```python
from build123d import *

# Parameters (mm, degrees)
BOSS_EXTRUDE1_DEPTH = 1.27
SKETCH2_R           = 2.0955
CUT_EXTRUDE1_DEPTH  = 2.27
CUT_EXTRUDE2_DEPTH  = 12.233456041


with BuildPart() as part:
    # Sketch1 → Boss-Extrude1 (new body)
    with BuildSketch(Plane.XY):
        with BuildLine():
            Line((48.63672497, 40.016070461), (47.23972497, 17.664070461))
            Line((47.23972497, 17.664070461), (45.08072497, 17.664070461))
            Line((45.08072497, 17.664070461), (45.138829135, 14.362070461))
            ThreePointArc((45.138829135, 14.362070461), (40.582766636, 12.764028795), (37.71472497, 16.648070461))
            Line((37.71472497, 16.648070461), (38.22272497, 23.760070461))
            ThreePointArc((38.22272497, 23.760070461), (38.367515348, 24.206944361), (38.746862194, 24.483994006))
            Line((38.746862194, 24.483994006), (39.635782378, 24.776070461))
            ThreePointArc((39.635782378, 24.776070461), (40.067551667, 25.379261916), (39.776898608, 26.061746677))
            ThreePointArc((39.776898608, 26.061746677), (38.984846047, 27.649488476), (39.74204727, 29.25414345))
            ThreePointArc((39.74204727, 29.25414345), (40.314007684, 29.599055552), (40.937994623, 29.360846875))
            ThreePointArc((40.937994623, 29.360846875), (42.372736858, 26.547570777), (44.82672497, 28.535270461))
            Line((44.82672497, 28.535270461), (44.82672497, 33.158070461))
            ThreePointArc((44.82672497, 33.158070461), (44.01481613, 36.330529444), (41.77872497, 38.722931645))
            Line((41.77872497, 38.722931645), (44.06472497, 45.350070461))
            Line((44.06472497, 45.350070461), (47.11272497, 45.350070461))
            Line((47.11272497, 45.350070461), (48.63672497, 40.016070461))
        make_face()
    extrude(amount=BOSS_EXTRUDE1_DEPTH)

    # Sketch2 → Cut-Extrude1 (cut, through all)
    with BuildSketch(Plane.XY.offset(1.27)):
        with Locations((41.77872497, 16.648070461)):
            Circle(SKETCH2_R)
    extrude(amount=-CUT_EXTRUDE1_DEPTH, mode=Mode.SUBTRACT)

    # Sketch3 → Cut-Extrude2 (cut, through all)
    with BuildSketch(Plane(origin=(45.956204144, -2.872262759, 0), x_dir=(0, 0, -1), z_dir=(0.998052578, -0.062378286, 0))):
        Polygon((-0.635, 48.200565798), (-1.27, 42.972017852), (-1.27, 48.200565798), align=None)
    extrude(amount=-CUT_EXTRUDE2_DEPTH, mode=Mode.SUBTRACT)


solid = part.part
```
Could you check a few things on this model? Use its own coordinates, in mm. A direction names the side the tool comes from. Coordinates: 2 decimals unless noted, no trailing zeros. Write each loop counter-clockwise with the first axis right and the second up, starting at its lowest first coordinate (ties: lowest second). Pieces come first, ordered by that corner, then holes. Notation, with made-up numbers: (-36, 12.25) -> (-15, 12.25) arc R30 ccw to (-15, 41.25) -> close; hole circle Ø10 at (-5, 9.25). An arc over 180 degrees is marked (long way). One line per question, with ' | ' between items. Start each with the question number.
1. If we section it at D-D (y = 23): Please give me the cut outline in (x, z).
2. Will this pin go through, and if not, where does the flat tip stop? P1, Ø6, axis at x = 43, y = 33, coming from the +Z side.
3. If we section it at B-B (x = 42.75): Please give me the cut outline in (y, z), and give its area (3 significant figures).
4. If we section it at C-C (x = 44.5): Please give me the cut outline in (y, z).
5. Please list where these lines run through material, in increasing order: line 1 along Y through (x, z) = (46.25, 0.4); line 2 along X through (y, z) = (17.5, 1.2); line 3 along X through (y, z) = (15.5, 0.4).
6. Thinking about a two-plate mould opening in Y: for faces 1 (the face through (40.652, 12.743, 0.626)), 2 (the face through (40.066, 25.368, 0.626)), 3 (the face through (40.304, 29.598, 0.626)), 4 (the face through (44, 26, 0)), which applies, pulls with the +Y half, pulls with the -Y half, needs draft (parallel to the pull), parting line crosses it, or undercut?
7. If we section it at A-A (z = 0.95): Please give me the cut outline in (x, y).
8. For faces 5 (the face through (37.965, 20.154, 0.626)), 6 (the face through (44.037, 36.29, 0.626)), 7 (the face through (44.827, 31, 1)), which set-ups out of +Z, -Z, +X, -X, +Y, -Y let a thin tool reach every point of the face, with its end or its side?
Return value:
1) outline: (38.17, 0) -> (47.57, 0) -> (47.57, 1.27) -> (38.17, 1.27) -> close
2) P1: stops at z = 1.27
3) outline: (12.7, 0) -> (14.79, 0) -> (14.79, 1.27) -> (12.7, 1.27) -> close; (18.5, 0) -> (26.5, 0) -> (26.5, 1.27) -> (18.5, 1.27) -> close; (37.97, 0) -> (41.54, 0) -> (41.54, 1.13) -> (40.38, 1.27) -> (37.97, 1.27) -> close | area: 17.3 mm²
4) outline: (13.63, 0) -> (27.43, 0) -> (27.43, 1.27) -> (13.63, 1.27) -> close; (35.21, 0) -> (45.35, 0) -> (45.35, 0.65) -> (40.27, 1.27) -> (35.21, 1.27) -> close
5) line 1: y = 17.66 to 45.35 | line 2: x = 37.78 to 39.86, 43.69 to 45.08 | line 3: x = 37.88 to 40.03, 43.53 to 45.12
6) face 1: pulls with the -Y half | face 2: undercut | face 3: pulls with the +Y half | face 4: needs draft
7) outline: (37.71, 16.65) arc R4.06 ccw to (45.14, 14.36) -> (45.08, 17.66) -> (47.24, 17.66) -> (48.64, 40.02) -> (47.87, 42.7) -> (43.25, 42.99) -> (41.78, 38.72) arc R6.6 cw to (44.83, 33.16) -> (44.83, 28.54) arc R2.03 cw (long way) to (40.94, 29.36) arc R0.76 ccw to (39.74, 29.25) arc R2.03 ccw to (39.78, 26.06) arc R0.76 cw to (39.64, 24.78) -> (38.75, 24.48) arc R0.76 ccw to (38.22, 23.76) -> close; hole circle Ø4.19 at (41.78, 16.65)
8) face 5: +Z, -Z, -X, +Y | face 6: +Z, -Z, -X | face 7: +Z, -Z
